Geometry: final body of the model. Coordinates: model frame, mm. A direction names the side the tool comes from. Give positions to 0.01 mm unless a question says otherwise; leave off trailing zeros. Order: outer loops, then holes, each group sorted by start corner. A loop starts at its lowest first (then second) coordinate and runs counter-clockwise, first axis right, second up. Notation, with made-up numbers: (15.25, 3.25) - (74.25, 3.25) arc R15 ccw to (74.25, 14.25) - close; hole circle Ø10 at (61.25, 20). An arc over 180 degrees is marked (long way). Use one line per item in the form item = value.
from build123d import *

# Parameters (mm, degrees)
PAD_DEPTH       = 15
SKETCH001_R     = 2.625
POCKET_DEPTH    = 5
POCKET001_DEPTH = 10


with BuildPart() as part:
    # Sketch → Pad (new body)
    with BuildSketch(Plane.XZ):
        Polygon((-68.87526, -5.227487), (-68.87526, 4.772513), (51.12474, 4.772513), (51.12474, -0.227487), (81.12474, -0.227487), (81.12474, -5.227487), align=None)
    extrude(amount=PAD_DEPTH)

    # Sketch001 (on Face4 of Pad) → Pocket (cut)
    with BuildSketch(Plane(origin=(0, 0, -0.227487), x_dir=(-1, 0, 0), z_dir=(0, 0, 1))):
        with Locations((-74.12474, 7.5)):
            Circle(SKETCH001_R)
        with Locations((-58.12474, 7.5)):
            Circle(SKETCH001_R)
    extrude(amount=-POCKET_DEPTH, mode=Mode.SUBTRACT)

    # Sketch002 (on Face3 of Pocket) → Pocket001 (cut)
    with BuildSketch(Plane(origin=(0, 0, 4.772513), x_dir=(-1, 0, 0), z_dir=(0, 0, 1))):
        Polygon((56.37526, 20.490381), (63.87526, 7.5), (48.87526, 7.5), align=None)
    extrude(amount=-POCKET001_DEPTH, mode=Mode.SUBTRACT)


solid = part.part
(1) Reachability of faces 1 (the face through (-61.68, -11.3, -0.16)), 2 (the face through (66, -7, -0.227)), 3 (the face through (7, 0, 0)) from +Z, -Z, +X, -X, +Y, -Y: full face, straight path, thin tool, end or side. Return the list, or none.
Computed values:
face_1 = +Z, -Z
face_2 = +Z, +X, +Y, -Y
face_3 = +Z, -Z, +X, -X, +Y
(2) Ray query, line 1 along X through (y, z) = (-8.25, -0.75); line 2 along X through (y, z) = (-8, -2.5); line 3 along Y through (x, z) = (-58, 3.5). Return the intervals inside material, ascending.
Computed values:
line_1 = -68.88 to -63.44, -49.31 to 55.61, 60.64 to 71.61, 76.64 to 81.12
line_2 = -68.88 to -63.59, -49.16 to 55.55, 60.7 to 71.55, 76.7 to 81.12
line_3 = -7.5 to 0
(3) Cut plane B-B on y = -11.5. Output: boundary loops of the cut face in (x, z), plus the area to 3 significant figures.
Computed values:
outline = (-68.88, -5.23) - (-61.57, -5.23) - (-61.57, 4.77) - (-68.88, 4.77) - close; (-51.18, -5.23) - (81.12, -5.23) - (81.12, -0.23) - (51.12, -0.23) - (51.12, 4.77) - (-51.18, 4.77) - close
area = 1,250 mm²
(4) Pull-direction query (X, two-part tool) for faces 4 (the face through (7, -7, -5.227)), 5 (the face through (-51.01, -11.2, -0.16)), 6 (the face through (51.125, -7, 2)); classes: released by +X, released by -X, zero draft, split by the parting line, or undercut.
Computed values:
face_4 = zero draft
face_5 = undercut
face_6 = released by +X
(5) Cut plane A-A on z = 1.25. Output: boundary loops of the cut face in (x, y).
Computed values:
outline = (-68.88, -15) - (-59.55, -15) - (-63.88, -7.5) - (-48.88, -7.5) - (-53.21, -15) - (51.12, -15) - (51.12, 0) - (-68.88, 0) - close
(6) Contact query for flat-ended pins moving along their axis: pin 1 Ø3 at (x, y) = (74.12, -7.5) entering from +Z; pin 2 Ø3 at (x, z) = (-55, 1.5) entering from -Y; pin 3 Ø4 at (y, z) = (-9.5, 3.5) entering from +X. Output: stop coordinate, or through.
Computed values:
pin_1 = through
pin_2 = -7.5
pin_3 = 51.12
